```python
from build123d import *

# Parameters (mm, degrees)
BOSS_EXTRUDE1_DEPTH = 3.5
SKETCH2_W           = 15
SKETCH2_H           = 15
CUT_EXTRUDE1_DEPTH  = 1
BOSS_EXTRUDE2_DEPTH = 20
BOSS_EXTRUDE3_DEPTH = 20
BOSS_EXTRUDE4_DEPTH = 20
SKETCH7_R           = 2
CUT_EXTRUDE3_DEPTH  = 20
SKETCH8_R           = 2
CUT_EXTRUDE4_DEPTH  = 20
SKETCH9_R           = 2
CUT_EXTRUDE5_DEPTH  = 20
SKETCH10_R          = 2
CUT_EXTRUDE6_DEPTH  = 20


with BuildPart() as part:
    # Sketch1 → Boss-Extrude1 (new body)
    with BuildSketch(Plane(origin=(0, 0, 0), x_dir=(1, 0, 0), z_dir=(0, 1, 0))):
        with BuildLine():
            Line((8, -10), (-8, -10))
            ThreePointArc((-8, -10), (-9.414213562, -9.414213562), (-10, -8))
            Line((-10, -8), (-10, 8))
            ThreePointArc((-10, 8), (-9.414213562, 9.414213562), (-8, 10))
            Line((-8, 10), (8, 10))
            ThreePointArc((8, 10), (9.414213562, 9.414213562), (10, 8))
            Line((10, 8), (10, -8))
            ThreePointArc((10, -8), (9.414213562, -9.414213562), (8, -10))
        make_face()
    extrude(amount=BOSS_EXTRUDE1_DEPTH)

    # Sketch2 → Cut-Extrude1 (cut)
    with BuildSketch(Plane(origin=(0, 3.5, 0), x_dir=(1, 0, 0), z_dir=(0, 1, 0))):
        with Locations((1, -1)):
            Rectangle(SKETCH2_W, SKETCH2_H)
    extrude(amount=-CUT_EXTRUDE1_DEPTH, mode=Mode.SUBTRACT)

    # Sketch3 → Boss-Extrude2 (add)
    with BuildSketch(Plane(origin=(0, 3.5, 0), x_dir=(1, 0, 0), z_dir=(0, 1, 0))):
        Polygon((2.803245497, 6.5), (-2.803245497, 6.5), (-5, 8.037515228), (-5, 8.537515228), (-3, 8.537515228), (-3, 10), (3, 10), (3, 8.537515228), (5, 8.537515228), (5, 8.037515228), align=None)
        Polygon((-8.537515228, 5), (-8.037515228, 5), (-6.5, 2.803245497), (-6.5, -2.803245497), (-8.037515228, -5), (-8.537515228, -5), (-8.537515228, -3), (-10, -3), (-10, 3), (-8.537515228, 3), align=None)
    extrude(amount=BOSS_EXTRUDE2_DEPTH)

    # Sketch4 → Boss-Extrude3 (add)
    with BuildSketch(Plane.XY.offset(10)):
        Polygon((2.93267729, 3.5), (4.950797873, 2), (4.950797873, 1.5), (3, 1.5), (3, 0), (-3, 0), (-3, 1.5), (-5.049202127, 1.5), (-5.049202127, 2), (-3.031081545, 3.5), align=None)
    extrude(amount=BOSS_EXTRUDE3_DEPTH)

    # Sketch5 → Boss-Extrude4 (add)
    with BuildSketch(Plane(origin=(10, 0, 0), x_dir=(0, 0, -1), z_dir=(1, 0, 0))):
        Polygon((2.803245497, 3.5), (5, 1.925227615), (5, 1.425227615), (3, 1.425227615), (3, 0), (-3, 0), (-3, 1.425227615), (-5, 1.425227615), (-5, 1.925227615), (-2.803245497, 3.5), align=None)
    extrude(amount=BOSS_EXTRUDE4_DEPTH)

    # Sketch7 → Cut-Extrude3 (cut)
    with BuildSketch(Plane.ZY.offset(10)):
        with Locations((0, 17.5)):
            Circle(SKETCH7_R)
    extrude(amount=-CUT_EXTRUDE3_DEPTH, mode=Mode.SUBTRACT)

    # Sketch8 → Cut-Extrude4 (cut)
    with BuildSketch(Plane(origin=(0, 0, -10), x_dir=(-1, 0, 0), z_dir=(0, 0, -1))):
        with Locations((0, 17.5)):
            Circle(SKETCH8_R)
    extrude(amount=-CUT_EXTRUDE4_DEPTH, mode=Mode.SUBTRACT)

    # Sketch9 → Cut-Extrude5 (cut)
    with BuildSketch(Plane(origin=(0, 3.5, 0), x_dir=(1, 0, 0), z_dir=(0, 1, 0))):
        with Locations(Location((0, -24, 0), (0, 0, 270))):
            Circle(SKETCH9_R)
    extrude(amount=-CUT_EXTRUDE5_DEPTH, mode=Mode.SUBTRACT)

    # Sketch10 → Cut-Extrude6 (cut)
    with BuildSketch(Plane(origin=(0, 3.5, 0), x_dir=(1, 0, 0), z_dir=(0, 1, 0))):
        with Locations(Location((24, 0, 0), (0, 0, 270))):
            Circle(SKETCH10_R)
    extrude(amount=-CUT_EXTRUDE6_DEPTH, mode=Mode.SUBTRACT)


solid = part.part
```
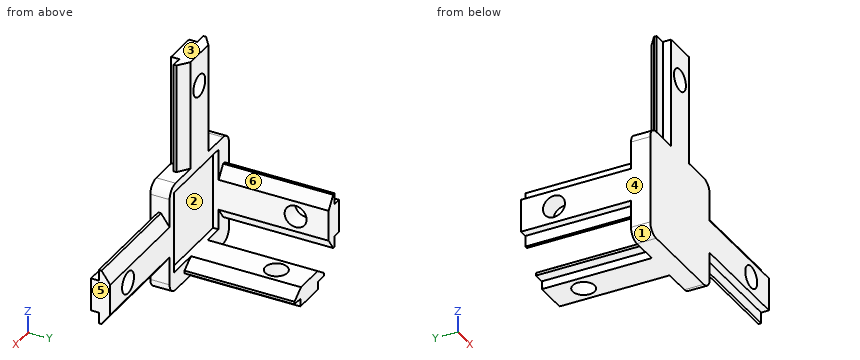
Model file for the job. Use its own axes, mm. Face numbers are marked on the shaded views. A direction names the side the tool comes from. Round coordinates to 2 decimals unless told otherwise and drop trailing zeros. Write each loop counter-clockwise with the first axis right and the second up, starting at its lowest first coordinate (ties: lowest second). Pieces come first, ordered by that corner, then holes. Notation, with made-up numbers: (40, 53.5) - (50, 53.5) arc R20 cw to (50, 86.5) - close; hole circle Ø11 at (57.25, -6). An arc over 180 degrees is marked (long way). Use CSV: the item, a comma, the result in double quotes. Start each with the question number.
Item 1: Drill centre lines: L1, parallel to X at y = 2.7, z = 0; L2, parallel to X at y = 2.25, z = 0; L3, parallel to X at y = 3.25, z = 3.5. Where is each one in solid material? Low to high. Write a range as [from, to].
Item 2: Band-saw the part on C-C (x = 24). Write the cut outline in (y, z).
Item 3: Two-plate mould, pull along Z, no slides. Class the marked faces 1, 2, 3 and 4: released by +Z, released by -Z, zero draft, split by the parting line, or undercut.
Item 4: Band-saw the part on B-B (y = 17.5). Write the cut outline in (x, z).
Item 5: Pin check, flat tips, straight feed: P1, Ø1.6, axis at x = -4, y = 14, coming from the -Z side; P2, Ø1.2, axis at x = -9, y = 17, coming from the +Z side; P3, Ø0.6, axis at y = 1.5, z = 25, coming from the -X side. Stop position of each tip, or through.
Item 6: Tool access for the marked faces 5 and 6: list every direction of +Z, -Z, +X, -X, +Y, -Y with a clear straight run to the whole face (end or side of a thin tool).
Item 7: Band-saw the part on D-D (z = 24). Write the cut outline in (x, y), and give its area (3 significant figures).
Item 8: Band-saw the part on A-A (z = 0). Write the cut outline in (x, y).
Checked values:
1,L1,"x = [-10, -6.5], [8.5, 22], [26, 30]"
1,L2,"x = [-10, 22], [26, 30]"
1,L3,"x = [-10, -6.5], [8.5, 10]"
2,outline,"(0, -3) - (1.43, -3) - (1.43, -5) - (1.93, -5) - (3.5, -2.8) - (3.5, -2) - (0, -2) - close; (0, 2) - (3.5, 2) - (3.5, 2.8) - (1.93, 5) - (1.43, 5) - (1.43, 3) - (0, 3) - close"
3,face 1,"released by -Z"
3,face 2,"undercut"
3,face 3,"released by +Z"
3,face 4,"zero draft"
4,outline,"(-10, -3) - (-8.54, -3) - (-8.54, -5) - (-8.04, -5) - (-6.5, -2.8) - (-6.5, -2) - (-10, -2) - close; (-10, 2) - (-6.5, 2) - (-6.5, 2.8) - (-8.04, 5) - (-8.54, 5) - (-8.54, 3) - (-10, 3) - close; (-5, -8.54) - (-3, -8.54) - (-3, -10) - (-2, -10) - (-2, -6.5) - (-2.8, -6.5) - (-5, -8.04) - close; (2, -10) - (3, -10) - (3, -8.54) - (5, -8.54) - (5, -8.04) - (2.8, -6.5) - (2, -6.5) - close"
5,P1,"stops at z = -8.54"
5,P2,"stops at z = 5"
5,P3,"stops at x = -5.05"
6,face 5,"+Z, -Z, +X, +Y, -Y"
6,face 6,"+Z, +X, +Y"
7,outline,"(-5.05, 1.5) - (-3, 1.5) - (-3, 0) - (-2, 0) - (-2, 3.5) - (-3.03, 3.5) - (-5.05, 2) - close; (2, 0) - (3, 0) - (3, 1.5) - (4.95, 1.5) - (4.95, 2) - (2.93, 3.5) - (2, 3.5) - close"
7,area,"12.0 mm²"
8,outline,"(-10, 0) - (22, 0) - (22, 3.5) - (8.5, 3.5) - (8.5, 2.5) - (-6.5, 2.5) - (-6.5, 15.5) - (-10, 15.5) - close; (-10, 19.5) - (-6.5, 19.5) - (-6.5, 23.5) - (-10, 23.5) - close; (26, 0) - (30, 0) - (30, 3.5) - (26, 3.5) - close"
